The figure shows three views and two pictorial views of one solid part (mm, origin at its lowest corner). Answer the questions. Coordinates: 2 decimals unless noted, no trailing zeros. Write each loop counter-clockwise with the first axis right and the second up, starting at its lowest first coordinate (ties: lowest second). Pieces come first, ordered by that corner, then holes. Notation, with made-up numbers: M -18,75.25 L -7,75.25 A19 ccw -7,112.25 Z; hole C 63.5,77 d8. An arc over 180 degrees is marked long. Use a Markdown table: item, result. Add a question column.
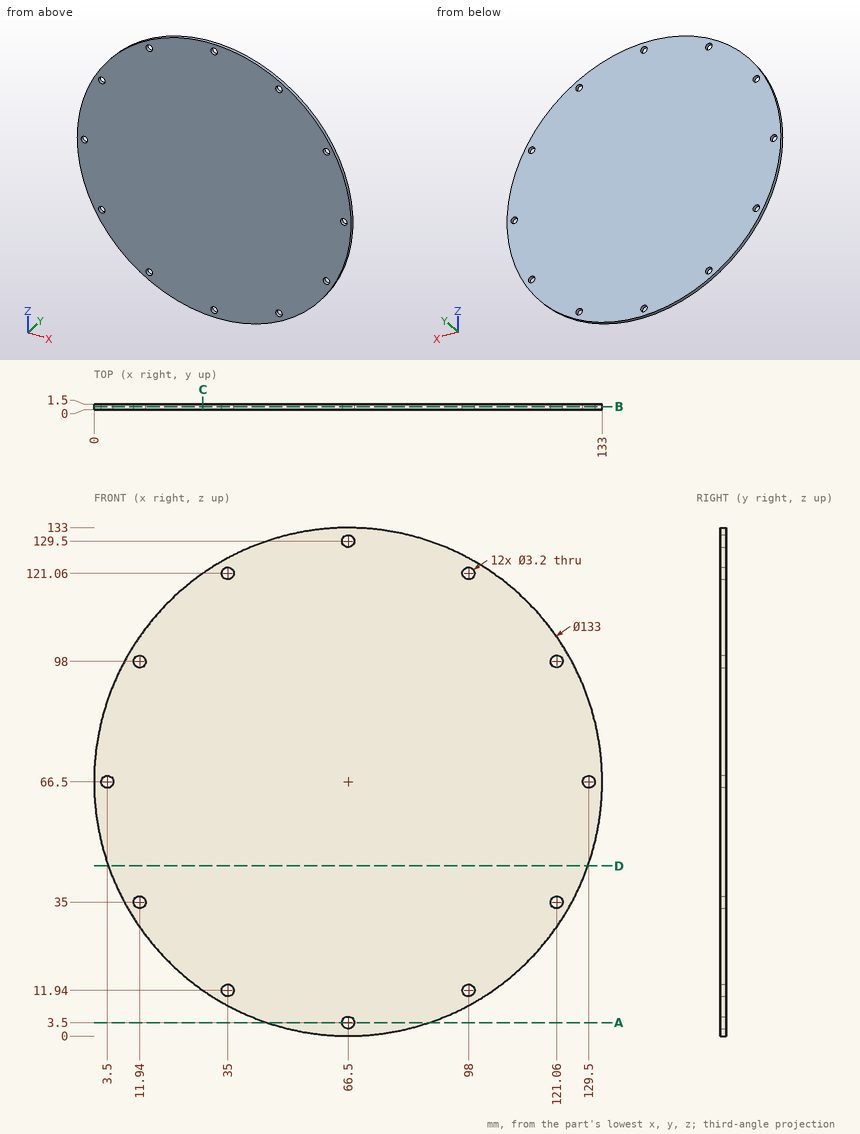
Item 1: Find section B-B on y = 0.8. Count the separate pieces of the cut face and the enclosed holes in it, then the cut area to 3 significant figures.
Item 2: Find section D-D on z = 44.5. Give the vertices of the cut face in (x, y) (1 decimal).
Item 3: This flat-tipped pin is pushed along its axis until it touches: pin 1 (4 mm diameter, centred on x = 129.5, z = 66.5, fed in from -Y). Where does it stop, or does it pass through?
Item 4: Consider probe 1 along Z at (x, y) = (66.5, 0.75); probe 2 along X at (y, z) = (0.4, 35) (1 decimal). Determine where each line is inside the solid, lowest interval first.
Item 5: Find section A-A on z = 3.5. Give the vertices of the cut face in (x, y).
Item 6: Find section C-C on x = 28.5. Give the vertices of the cut face in (y, z).
Geometry says:
| question | item | result |
|---|---|---|
| 1 | separate pieces | 1 |
| 1 | enclosed holes | 12 |
| 1 | area | 13,800 mm2 |
| 2 | outline | M 3.7,0 L 129.3,0 L 129.3,1.5 L 3.7,1.5 Z |
| 3 | pin 1 | stops at y = 0 |
| 4 | probe 1 | z = 0 to 1.9, 5.1 to 127.9, 131.1 to 133 |
| 4 | probe 2 | x = 7.9 to 10.3, 13.5 to 119.5, 122.7 to 125.1 |
| 5 | outline | M 45.21,0 L 64.9,0 L 64.9,1.5 L 45.21,1.5 Z; M 68.1,0 L 87.79,0 L 87.79,1.5 L 68.1,1.5 Z |
| 6 | outline | M 0,11.93 L 1.5,11.93 L 1.5,121.07 L 0,121.07 Z |
